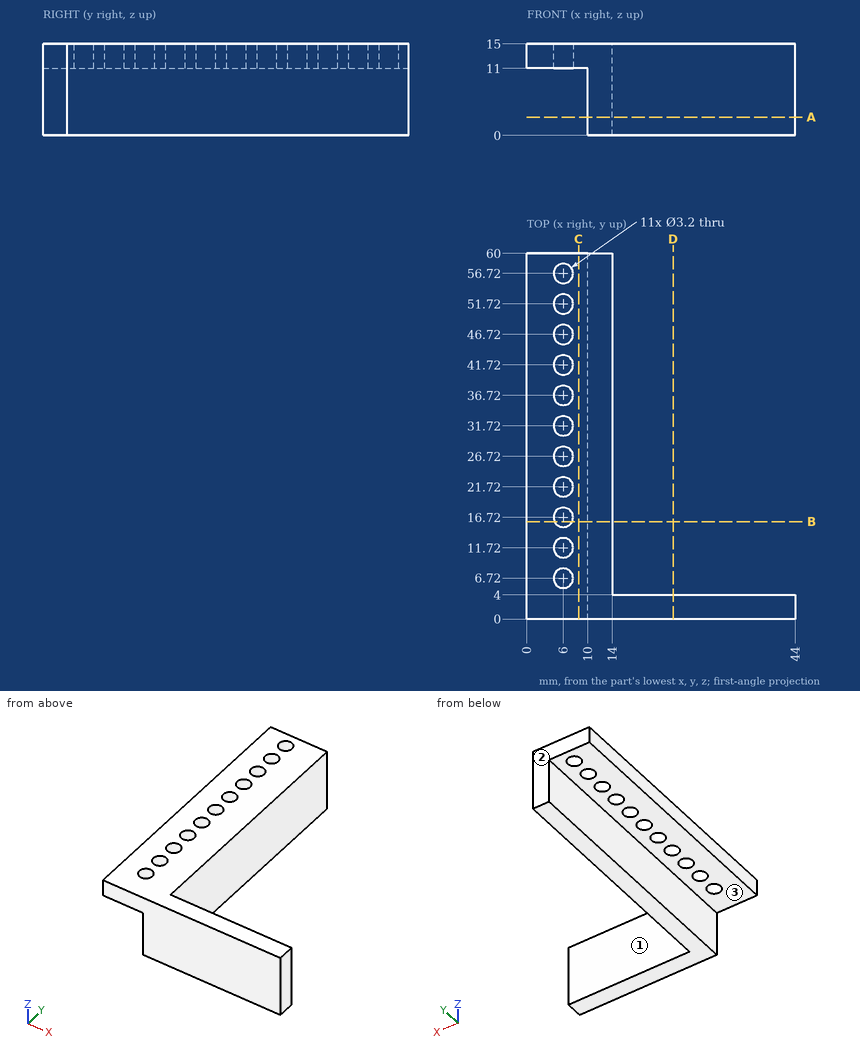
Answer from the drawing. Dimensions are ordinates in mm from the lowest x, y and z of the part. A direction names the side the tool comes from. Coordinates: 2 decimals unless noted, no trailing zeros. Write each loop counter-clockwise with the first axis right and the second up, starting at its lowest first coordinate (ties: lowest second). Pieces come first, ordered by that corner, then holes. Notation, with made-up numbers: (36, 44) - (72, 44) arc R26 ccw to (72, 74) - close; hole circle Ø10 at (39.25, 15.5). An arc over 180 degrees is marked (long way). Return JSON: item names as keys, results as strings. Group by question number.
Q1. The part is cut by section B-B on y = 16. Write down the section's boundary in (x, z).
Q2. The part is cut by section D-D on x = 24. Write down the section's boundary in (y, z), and give its area (3 significant figures).
Q3. Find the intervals of material crossed by line 1 along X through (y, z) = (23.5, 14.25); line 2 along X through (y, z) = (21, 6); line 3 along X through (y, z) = (22, 12.25) (1 decimal), in increasing order. Write a range as [from, to].
Q4. Flat-ended cylindrical pins translate along their axes: pin 1 Ø9 at (y, z) = (27.5, 5.5) entering from -X; pin 2 Ø3 at (x, y) = (4.5, 27.5) entering from -Z; pin 3 Ø1.5 at (y, z) = (29, 2) entering from +X. Find the tip coordinate at first contact, or state that the pin passes through.
Q5. The part is cut by section A-A on z = 3. Write down the section's boundary in (x, y), and give its area (3 significant figures).
Q6. Which of the six approach directions +Z, -Z, +X, -X, +Y, -Y give full straight-line access (tool end or side, diameter ignored) to the marked faces 1, 2 and 3?
Q7. The part is cut by section C-C on x = 8.5. Write down the section's boundary in (y, z).
Evaluation:
{
 "1": {"outline": "(0, 11) - (4.57, 11) - (4.57, 15) - (0, 15) - close; (7.43, 11) - (10, 11) - (10, 0) - (14, 0) - (14, 15) - (7.43, 15) - close"},
 "2": {"outline": "(0, 0) - (4, 0) - (4, 15) - (0, 15) - close", "area": "60.0 mm2"},
 "3": {"line 1": "x = [0, 14]", "line 2": "x = [10, 14]", "line 3": "x = [0, 4.4], [7.6, 14]"},
 "4": {"pin 1": "stops at x = 10", "pin 2": "stops at z = 11", "pin 3": "stops at x = 14"},
 "5": {"outline": "(10, 0) - (44, 0) - (44, 4) - (14, 4) - (14, 60) - (10, 60) - close", "area": "360 mm2"},
 "6": {"face 1": "+Z, -Z, +X, +Y", "face 2": "+Z, -Z, +X, -X, +Y", "face 3": "-Z, -X, +Y, -Y"},
 "7": {"outline": "(0, 11) - (60, 11) - (60, 15) - (0, 15) - close"}
}
